from build123d import *

# Parameters (mm, degrees)
BOSS_EXTRUDE1_DEPTH     = 36
CUT_EXTRUDE1_DEPTH      = 175.416168975
CUT_EXTRUDE1_DEPTH_BACK = 10
SKETCH2_R               = 30
SKETCH3_W               = 72
SKETCH3_H               = 38.639129372
CUT_EXTRUDE2_DEPTH      = 10
SKETCH4_R               = 12
CUT_EXTRUDE3_DEPTH      = 167.195667814
SKETCH5_W               = 50
SKETCH5_H               = 5
CUT_EXTRUDE4_DEPTH      = 70
CUT_EXTRUDE5_DEPTH      = 70


with BuildPart() as part:
    # Sketch1 → Boss-Extrude1 (new, symmetric)
    with BuildSketch(Plane(origin=(0, 0, 0), x_dir=(-1, 0, 0), z_dir=(0, 1, 0))):
        Polygon((0, 0), (145, 0), (145, 25), (35, 25), (35, 90), (0, 90), align=None)
    extrude(amount=BOSS_EXTRUDE1_DEPTH, both=True)

    # Sketch2 → Cut-Extrude1 (cut, two sides: drawn at the far end of the back side and taken through both)
    with BuildSketch(Plane.YZ.offset(-CUT_EXTRUDE1_DEPTH_BACK)):
        with Locations(Location((0, 45, 0), (0, 0, 90))):
            Circle(SKETCH2_R)
    extrude(amount=CUT_EXTRUDE1_DEPTH + CUT_EXTRUDE1_DEPTH_BACK, mode=Mode.SUBTRACT)

    # Sketch3 → Cut-Extrude2 (cut)
    with BuildSketch(Plane.YZ):
        with Locations((0, 46.680435314)):
            Rectangle(SKETCH3_W, SKETCH3_H)
    extrude(amount=-CUT_EXTRUDE2_DEPTH, mode=Mode.SUBTRACT)

    # Sketch4 → Cut-Extrude3 (cut, through all)
    with BuildSketch(Plane.YZ.offset(-10)):
        with Locations(Location((0, 45, 0), (0, 0, 270))):
            Circle(SKETCH4_R)
    extrude(amount=-CUT_EXTRUDE3_DEPTH, mode=Mode.SUBTRACT)

    # Sketch5 → Cut-Extrude4 (cut)
    with BuildSketch(Plane.YZ):
        with Locations((11, 2.5)):
            Rectangle(SKETCH5_W, SKETCH5_H)
    extrude(amount=-CUT_EXTRUDE4_DEPTH, mode=Mode.SUBTRACT)

    # Sketch6 → Cut-Extrude5 (cut)
    with BuildSketch(Plane.XY.offset(25)):
        with BuildLine():
            Line((-95, 12), (-145, 12))
            Line((-145, 12), (-145, -12))
            Line((-145, -12), (-95, -12))
            ThreePointArc((-95, -12), (-83, 0), (-95, 12))
        make_face()
    extrude(amount=-CUT_EXTRUDE5_DEPTH, mode=Mode.SUBTRACT)


solid = part.part
CAD build for the part. Positions are in the model's coordinates, mm. A direction names the side the tool comes from. Give positions to 0.01 mm unless a question says otherwise; leave off trailing zeros. Write each loop counter-clockwise with the first axis right and the second up, starting at its lowest first coordinate (ties: lowest second). Pieces come first, ordered by that corner, then holes. Notation, with made-up numbers: (-1, -12.5) - (15, -12.5) arc R28 cw to (15, 11.5) - close; hole circle Ø6 at (28, 5). An arc over 180 degrees is marked (long way). Put each result on its own line as item: value.
(1) Pull direction Y, two halves, no side cores. Call faces 1 (the flat face through (-35, -14, 2)), 2 (the cylindrical face through (-5, 0, 15)), 3 (the flat face through (-71, -7, 0)), 4 (the cylindrical face through (-22.32, 0.53, 56.99)): released by +Y, released by -Y, zero draft, split by the parting line, or undercut.
Working result:
face 1: released by +Y
face 2: undercut
face 3: zero draft
face 4: undercut
(2) Saw through at D-D (y = 29.5). List the corners of the cut face in (x, z).
Working result:
outline: (-145, 0) - (-70, 0) - (-70, 5) - (0, 5) - (0, 27.36) - (-10, 27.36) - (-10, 66) - (0, 66) - (0, 90) - (-35, 90) - (-35, 25) - (-145, 25) - close
(3) Tool access for faces 5 (the flat face through (-35, 11, 5)), 6 (the flat face through (-5, 29, 66)), 7 (the flat face through (-35, 1, 64)): list every direction of +Z, -Z, +X, -X, +Y, -Y with a clear straight run to the whole face (end or side of a thin tool).
Working result:
face 5: -Z, +X, +Y
face 6: +X, +Y, -Y
face 7: +Z, -X, +Y, -Y
(4) Wall check: L1, parallel to Y at x = -24, z = 45; L2, parallel to Z at x = -115, y = -16.5; L3, parallel to X at y = 16.5, z = 35.5. Give the ranges that are in metal, low to high.
Working result:
L1: -36 to -12, 12 to 36
L2: 0 to 25
L3: -35 to -10
(5) Saw through at B-B (z = 45). List the corners of the cut face in (x, y).
Working result:
outline: (-35, -36) - (-10, -36) - (-10, -12) - (-35, -12) - close; (-35, 12) - (-10, 12) - (-10, 36) - (-35, 36) - close
(6) Saw through at C-C (x = -98). List the corners of the cut face in (y, z).
Working result:
outline: (-36, 0) - (-12, 0) - (-12, 25) - (-36, 25) - close; (12, 0) - (36, 0) - (36, 25) - (12, 25) - close
(7) Drop flat-ended pins along their axis: pin 1 Ø1.5 at (y, z) = (27.5, 63.5) entering from +X; pin 2 Ø19.5 at (y, z) = (-12.5, 44.5) entering from -X; pin 3 Ø8 at (x, y) = (-3.5, 26.5) entering from -Z; pin 4 Ø19 at (y, z) = (0, 45) entering from -X. Give the stop position or say it passes through.
Working result:
pin 1: x = -10
pin 2: x = -35
pin 3: z = 5
pin 4: through
(8) Saw through at A-A (y = 0). List the corners of the cut face in (x, z), then the cut area to 3 significant figures.
Working result:
outline: (-83, 0) - (-70, 0) - (-70, 5) - (0, 5) - (0, 15) - (-10, 15) - (-10, 33) - (-35, 33) - (-35, 25) - (-83, 25) - close; (-35, 57) - (-10, 57) - (-10, 75) - (0, 75) - (0, 90) - (-35, 90) - close
area: 2,800 mm^2
